from build123d import *

# Parameters (mm, degrees)
EXTRUDE_1_DEPTH = 480
SCALE_1_SCALE   = 1.3


with BuildPart() as part:
    # 草图1 → 凸台-拉伸1 (new body)
    with BuildSketch(Plane.XY):
        with BuildLine():
            Line((-8442.584105349, 4688), (-7962.584105349, 4688))
            ThreePointArc((-7962.584105349, 4688), (-7883.943917736, 4831.891322342), (-7793.3126292, 4968.547684402))
            ThreePointArc((-7793.3126292, 4968.547684402), (-7737.474510483, 5041.653065761), (-7678.198873592, 5112))
            Line((-7678.198873592, 5112), (-8158.198873592, 5112))
            Line((-8158.198873592, 5112), (-8442.584105349, 5112))
            Line((-8442.584105349, 5112), (-8442.584105349, 4688))
        make_face()
    extrude(amount=EXTRUDE_1_DEPTH)


with BuildPart() as part_1:
    # 缩放比例1: scaled about (0, 0, 0)
    add(part.part.scale(SCALE_1_SCALE))


solid = part_1.part
Part model, mm, in its own coordinate system. Give positions to 0.01 mm unless a question says otherwise; leave off trailing zeros. Order: outer loops, then holes, each group sorted by start corner. A loop starts at its lowest first (then second) coordinate and runs counter-clockwise, first axis right, second up. Notation, with made-up numbers: (63, -32.75) -> (111, -32.75) arc R19 ccw to (111, -18.75) -> close; hole circle Ø5 at (61, 0.25). An arc over 180 degrees is marked (long way). Use one line per item in the form item = value.
(1) Saw through at A-A (z = 397.5). Write the cut outline in (x, y), then the cut area to 3 significant figures.
Solution:
outline = (-10975.36, 6094.4) -> (-10351.36, 6094.4) arc R2496 cw to (-9981.66, 6645.6) -> (-10975.36, 6645.6) -> close
area = 436,000 mm²
(2) Flat gauge pins, fed straight in: P1, Ø12, axis at y = 6467, z = 471.5, coming from the +X side; P2, Ø12, axis at y = 6314, z = 512.5, coming from the +X side; P3, Ø10, axis at x = -10088.5, z = 184, coming from the -Y side. Where does each tip first touch, or does it go through?
Solution:
P1 = -10121.14
P2 = -10225.39
P3 = 6509.79
(3) Saw through at C-C (y = 6561). Write the cut outline in (x, z), then the cut area to 3 significant figures.
Solution:
outline = (-10975.36, 0) -> (-10053.2, 0) -> (-10053.2, 624) -> (-10975.36, 624) -> close
area = 575,000 mm²
(4) Saw through at B-B (x = -10203). Write the cut outline in (y, z).
Solution:
outline = (6354.99, 0) -> (6645.6, 0) -> (6645.6, 624) -> (6354.99, 624) -> close
(5) Drill centre lines: line 1 (Y direction, x = -10270, z = 514.5); line 2 (Y direction, x = -10110, z = 143); line 3 (X direction, y = 6371, z = 27). Where is each one in solid material? Low to high. Write a range as from..to.
Solution:
line_1 = 6246.21..6645.6
line_2 = 6488..6645.6
line_3 = -10975.36..-10192.47
